```python
from build123d import *

# Parameters (mm, degrees)
SKETCH_1_W               = 70
SKETCH_1_H               = 160.68
EXTRUDE_1_DEPTH          = 1.5
CUT_EXTRUDE_1_DEPTH      = 126.760303041
CUT_EXTRUDE_1_DEPTH_BACK = 126.760303041
SKETCH_2_R               = 2.2
FILLET_2_R               = 10
CUT_EXTRUDE_2_DEPTH      = 126.760303041
CUT_EXTRUDE_2_DEPTH_BACK = 126.760303041
SKETCH_3_R               = 2.2
CHAMFER_2_SIZE           = 40
CHAMFER_2_SIZE2          = 26.108145787
FILLET_3_R               = 5
CUT_EXTRUDE_3_DEPTH      = 112.92791923
CUT_EXTRUDE_3_DEPTH_BACK = 112.92791923
SKETCH_4_W               = 3.3
SKETCH_4_H               = 15.4
SKETCH_5_R               = 2.15
CUT_EXTRUDE_4_DEPTH      = 10


with BuildPart() as part:
    # 草图1 → 凸台-拉伸1 (new, symmetric)
    with BuildSketch(Plane(origin=(0, 0, 0), x_dir=(1, 0, 0), z_dir=(0, 1, 0))):
        Rectangle(SKETCH_1_W, SKETCH_1_H)
        Polygon((35, 80.34), (-35, 120.754518843), (-35, 80.34), align=None)
    extrude(amount=EXTRUDE_1_DEPTH, both=True)

    # 草图2 → 切除-拉伸1 (cut, two sides: drawn at the far end of the back side and taken through both)
    with BuildSketch(Plane(origin=(0, 1.5, 0), x_dir=(1, 0, 0), z_dir=(0, 1, 0)).offset(-CUT_EXTRUDE_1_DEPTH_BACK)):
        with Locations(Location((-12, 95.928457268, 0), (0, 0, 270))):
            Circle(SKETCH_2_R)
        with Locations(Location((17.444863729, 78.928457268, 0), (0, 0, 270))):
            Circle(SKETCH_2_R)
    extrude(amount=CUT_EXTRUDE_1_DEPTH + CUT_EXTRUDE_1_DEPTH_BACK, mode=Mode.SUBTRACT)

    # 圆角2
    fillet_2_edges = [part.edges().sort_by_distance(p)[0] for p in [
        (35, 0, -80.34),
    ]]
    fillet(fillet_2_edges, radius=FILLET_2_R)

    # 草图3 → 切除-拉伸2 (cut, two sides: drawn at the far end of the back side and taken through both)
    with BuildSketch(Plane(origin=(0, 1.5, 0), x_dir=(1, 0, 0), z_dir=(0, 1, 0)).offset(-CUT_EXTRUDE_2_DEPTH_BACK)):
        with Locations(Location((0, -70.34, 0), (0, 0, 270))):
            Circle(SKETCH_3_R)
        with Locations(Location((-20, -70.34, 0), (0, 0, 270))):
            Circle(SKETCH_3_R)
        with Locations(Location((20, -70.34, 0), (0, 0, 270))):
            Circle(SKETCH_3_R)
    extrude(amount=CUT_EXTRUDE_2_DEPTH + CUT_EXTRUDE_2_DEPTH_BACK, mode=Mode.SUBTRACT)

    # 倒角2
    chamfer_2_edges = [part.edges().sort_by_distance(p)[0] for p in [
        (-35, 0, -120.754518843),
    ]]
    chamfer_2_side = [part.faces().sort_by_distance(p)[0] for p in [
        (-35, 0, -20.207259422),
    ]]
    chamfer(chamfer_2_edges, length=CHAMFER_2_SIZE, length2=CHAMFER_2_SIZE2, reference=chamfer_2_side[0])

    # 圆角3
    fillet_3_edges = [part.edges().sort_by_distance(p)[0] for p in [
        (-35, 0, -80.754518843),
        (-12.389682503, 0, -107.70044595),
    ]]
    fillet(fillet_3_edges, radius=FILLET_3_R)

    # 草图4 → 切除-拉伸3 (cut, two sides: drawn at the far end of the back side and taken through both)
    with BuildSketch(Plane(origin=(0, 1.5, 0), x_dir=(1, 0, 0), z_dir=(0, 1, 0)).offset(-CUT_EXTRUDE_3_DEPTH_BACK)):
        with Locations((-27.35, -22.64)):
            Rectangle(SKETCH_4_W, SKETCH_4_H)
        with Locations((27.35, -32.64)):
            Rectangle(SKETCH_4_W, SKETCH_4_H)
        with Locations((27.35, 17.76)):
            Rectangle(SKETCH_4_W, SKETCH_4_H)
    extrude(amount=CUT_EXTRUDE_3_DEPTH + CUT_EXTRUDE_3_DEPTH_BACK, mode=Mode.SUBTRACT)

    # 草图5 → 切除-拉伸4 (cut)
    with BuildSketch(Plane(origin=(0, 1.5, 0), x_dir=(1, 0, 0), z_dir=(0, 1, 0))):
        with Locations(Location((-21.232050808, 83.938076211, 0), (0, 0, 270))):
            Circle(SKETCH_5_R)
        with Locations(Location((11.676914536, 64.938076211, 0), (0, 0, 270))):
            Circle(SKETCH_5_R)
    extrude(amount=-CUT_EXTRUDE_4_DEPTH, mode=Mode.SUBTRACT)


solid = part.part
```
Work out the finished part from the listing and answer in its coordinate system (mm). A direction names the side the tool comes from. Round coordinates to 2 decimals unless told otherwise and drop trailing zeros. Loops run counter-clockwise (first coordinate to the right, second up) from the corner with the lowest first, then second, coordinate; pieces in that order, holes last.
(1) Each of these flat-tipped pins is pushed along its axis until it touches: P1, Ø5, axis at x = -21.23, z = -83.94, coming from the -Y side; P2, Ø1, axis at y = 1, z = -84, coming from the +X side; P3, Ø1.5, axis at x = 27, y = 0.5, coming from the -Z side. Where does it stop, or does it pass through?
Computed values:
P1: stops at y = -1.5
P2: stops at x = 29.53
P3: stops at z = -85.39
(2) The part is cut by section C-C, the plane x = 0. Give the vertices of the cut face in (y, z), and give its area (3 significant figures).
Computed values:
outline: (-1.5, -100.55) - (1.5, -100.55) - (1.5, 68.14) - (-1.5, 68.14) - close; (-1.5, 72.54) - (1.5, 72.54) - (1.5, 80.34) - (-1.5, 80.34) - close
area: 529 mm2
(3) The part is cut by section B-B, the plane z = -18. Give the vertices of the cut face in (x, y).
Computed values:
outline: (-35, -1.5) - (25.7, -1.5) - (25.7, 1.5) - (-35, 1.5) - close; (29, -1.5) - (35, -1.5) - (35, 1.5) - (29, 1.5) - close
(4) The part is cut by section A-A, the plane z = 70.34. Give the vertices of the cut face in (x, y).
Computed values:
outline: (-35, -1.5) - (-22.2, -1.5) - (-22.2, 1.5) - (-35, 1.5) - close; (-17.8, -1.5) - (-2.2, -1.5) - (-2.2, 1.5) - (-17.8, 1.5) - close; (2.2, -1.5) - (17.8, -1.5) - (17.8, 1.5) - (2.2, 1.5) - close; (22.2, -1.5) - (35, -1.5) - (35, 1.5) - (22.2, 1.5) - close
(5) For faces 1 (the cylindrical face through (-12.1, 0, -106.2)), 2 (the flat face through (27, 0, 24.94)), determine the directions among +Z, -Z, +X, -X, +Y, -Y from which every point of the face is accessible in a straight line to the end or side of a thin tool.
Computed values:
face 1: -Z, +Y, -Y
face 2: +Y, -Y
(6) Find the intervals of material crossed by L1, parallel to X at y = 0.7, z = 70.34; L2, parallel to X at y = 0.15, z = 29; L3, parallel to X at y = -0.9, z = 31.5, in increasing order.
Computed values:
L1: x = -35 to -22.2, -17.8 to -2.2, 2.2 to 17.8, 22.2 to 35
L2: x = -35 to -29, -25.7 to 25.7, 29 to 35
L3: x = -35 to 25.7, 29 to 35
(7) The mould has two halves that part along Z. Classify faces 3 (the flat face through (0, 0, 80.34)), 4 (the cylindrical face through (18.11, -0.02, -76.83)), 5 (the flat face through (-24.33, 0.02, -93.47)): pulls with the +Z half, pulls with the -Z half, needs draft (parallel to the pull), parting line crosses it, or undercut.
Computed values:
face 3: pulls with the +Z half
face 4: undercut
face 5: pulls with the -Z half
(8) The part is cut by section D-D, the plane y = 0.1. Give the number of separate pieces and of enclosed holes in the cut face, and give its area (3 significant figures).
Computed values:
separate pieces: 1
enclosed holes: 10
area: 11,900 mm2
